Geometry check sheet. Reference: drawing and pictorial views, mm from the part's lowest x, y, z. A direction names the side the tool comes from. Give positions to 0.01 mm unless a question says otherwise; leave off trailing zeros. Order: outer loops, then holes, each group sorted by start corner. A loop starts at its lowest first (then second) coordinate and runs counter-clockwise, first axis right, second up. Notation, with made-up numbers: (-29.5, 51.5) - (4.5, 51.5) arc R20 cw to (4.5, 60.5) - close; hole circle Ø8 at (-3, 20.25). An arc over 180 degrees is marked (long way). Answer as a JSON object with one key per item and string values.
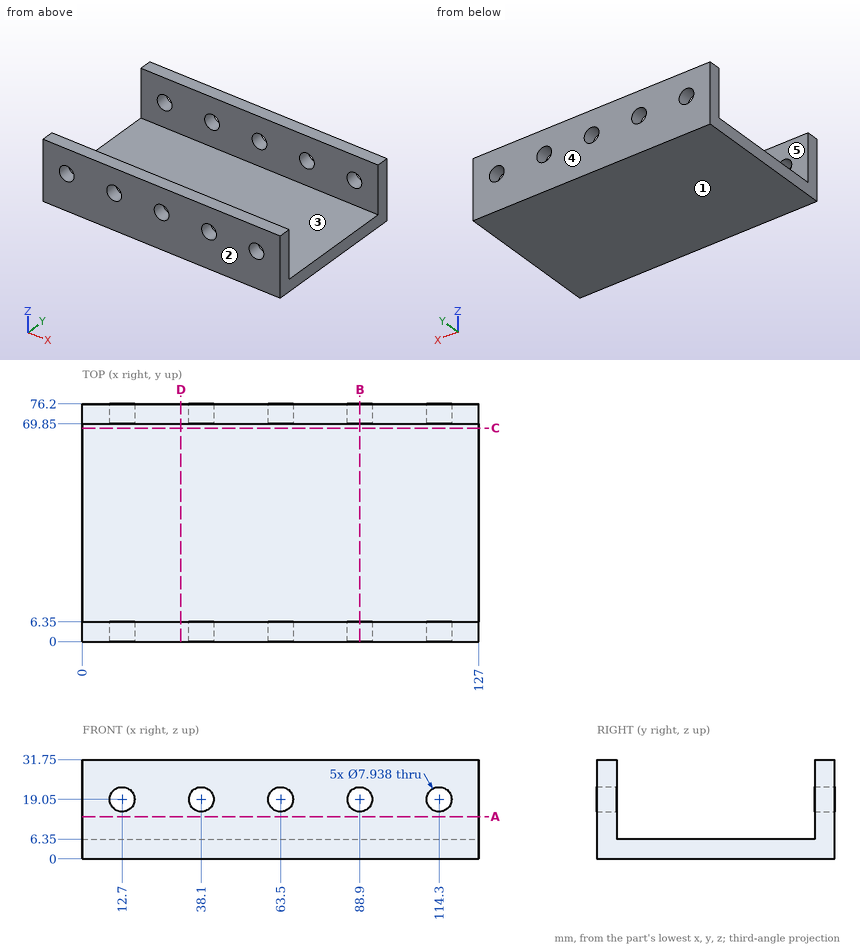
(1) Gauge pin test, flat end, axial feed: pin 1 Ø2 at (x, y) = (96, 55.5) entering from +Z. Record the tip position at first contact, or that the pin passes through.
Computed values:
{"pin 1": "stops at z = 6.35"}
(2) Section check C-C (y = 68.5). Record the cut outline in (x, z).
Computed values:
{"outline": "(0, 0) - (127, 0) - (127, 6.35) - (0, 6.35) - close"}
(3) Section check B-B (x = 88.9). Record the cut outline in (y, z).
Computed values:
{"outline": "(0, 0) - (76.2, 0) - (76.2, 15.08) - (69.85, 15.08) - (69.85, 6.35) - (6.35, 6.35) - (6.35, 15.08) - (0, 15.08) - close; (0, 23.02) - (6.35, 23.02) - (6.35, 31.75) - (0, 31.75) - close; (69.85, 23.02) - (76.2, 23.02) - (76.2, 31.75) - (69.85, 31.75) - close"}
(4) Access from +Z, -Z, +X, -X, +Y, -Y to the whole of each face (thin tool, end or side, straight path). Record for the marked faces 4 and 5.
Computed values:
{"face 4": "+Z, -Z, +X, -X, +Y", "face 5": "+Z, +X, -X"}
(5) Section check A-A (z = 13.5). Record the cut outline in (x, y), then the cut area to 3 significant figures.
Computed values:
{"outline": "(0, 0) - (127, 0) - (127, 6.35) - (0, 6.35) - close; (0, 69.85) - (127, 69.85) - (127, 76.2) - (0, 76.2) - close", "area": "1,610 mm²"}
(6) Material ranges on line 1 along X through (y, z) = (72, 19); line 2 along Y through (x, z) = (117, 28); line 3 along Z through (x, y) = (12.7, 4), recorded low to high. Write a range as [from, to].
Computed values:
{"line 1": "x = [0, 8.73], [16.67, 34.13], [42.07, 59.53], [67.47, 84.93], [92.87, 110.33], [118.27, 127]", "line 2": "y = [0, 6.35], [69.85, 76.2]", "line 3": "z = [0, 15.08], [23.02, 31.75]"}
(7) Release check for a two-part mould opening along Y. For the marked faces 1, 2 and 3 record: pulls with the +Y half, pulls with the -Y half, needs draft (parallel to the pull), parting line crosses it, or undercut.
Computed values:
{"face 1": "needs draft", "face 2": "pulls with the -Y half", "face 3": "undercut"}
(8) Section check D-D (x = 31.5). Record the cut outline in (y, z).
Computed values:
{"outline": "(0, 0) - (76.2, 0) - (76.2, 31.75) - (69.85, 31.75) - (69.85, 6.35) - (6.35, 6.35) - (6.35, 31.75) - (0, 31.75) - close"}
